The model under review builds one solid part; all positions refer to its coordinate system, in mm. Face numbers are marked on the shaded views. A direction names the side the tool comes from. Coordinates: 2 decimals unless noted, no trailing zeros. Order: outer loops, then holes, each group sorted by start corner. A loop starts at its lowest first (then second) coordinate and runs counter-clockwise, first axis right, second up. Notation, with made-up numbers: (39.25, 60) -> (65.25, 60) arc R18 cw to (65.25, 93) -> close; hole circle Ø9 at (-27, 26). An arc over 180 degrees is marked (long way). Use one line per item in the form item = value.
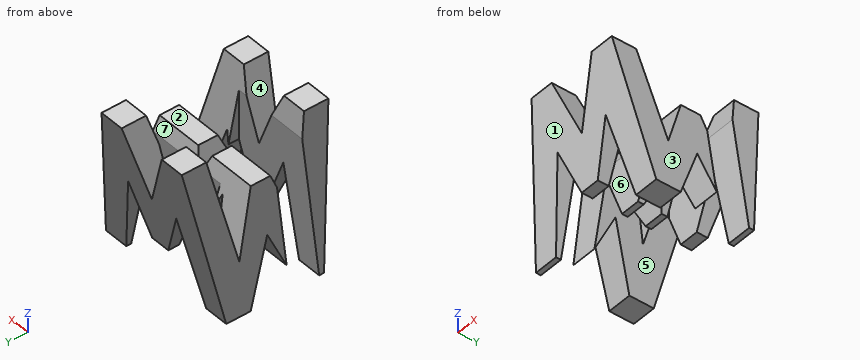
from build123d import *

# Parameters (mm, degrees)
F0_W      = 38.1
F0_H      = 38.1
F1_DEPTH  = 38.1
F6_DEPTH  = 38.1
F8_DEPTH  = 38.1
F9_W      = 25.4
F9_H      = 7.62
F10_DEPTH = 38.1


# Not quite as in the source:
# - a feature names something its author has since deleted; it is built from what else it names


with BuildPart() as f1:
    # F0 (on Front) → F1 (new body)
    with BuildSketch(Plane.XZ):
        with Locations((19.05, 19.05)):
            Rectangle(F0_W, F0_H)
    extrude(amount=F1_DEPTH)

    # F5 (on offset) → F6 (cut)
    with BuildSketch(Plane.YZ.offset(38.1)):
        Polygon((-11.43, 12.2219994664), (-6.35, 38.1), (-31.75, 38.1), (-26.67, 14.2379999161), (-21.59, 27.6940000847), (-16.51, 27.6940000847), align=None)
        Polygon((-31.75, 0), (-38.1, 38.1), (-38.1, 0), align=None)
        Polygon((-25.4, 0), (-19.05, 0), (-19.05, 14.9940000847), align=None)
        Polygon((-19.05, 0), (-12.7, 0), (-19.05, 14.9940000847), align=None)
        Polygon((-6.35, 0), (0, 0), (0, 38.1), align=None)
    extrude(amount=-F6_DEPTH, mode=Mode.SUBTRACT)

    # F7 (on offset) → F8 (cut)
    with BuildSketch(Plane.XZ.offset(38.1)):
        Polygon((0, 38.1), (0, 0), (6.35, 38.1), align=None)
        Polygon((25.4, 38.1), (12.7, 38.1), (19.05, 22.225), align=None)
        Polygon((31.75, 38.1), (38.1, 0), (38.1, 38.1), align=None)
        Polygon((11.340001598, 22.225), (6.35, 0), (31.660001598, 0), (26.580001598, 22.2758815411), (21.500001598, 9.525), (16.420001598, 9.525), align=None)
    extrude(amount=-F8_DEPTH, mode=Mode.SUBTRACT)

    # F9 (on offset) → F10 (cut)
    with BuildSketch(Plane.XY.offset(38.1)):
        with Locations((25.4, -11.43)):
            Rectangle(F9_W, F9_H)
        with Locations((12.7, -26.67)):
            Rectangle(F9_W, F9_H)
    extrude(amount=-F10_DEPTH, mode=Mode.SUBTRACT)


solid = f1.part
Item 1: We need section B-B (z = 23). State how many separate pieces and enclosed holes the cut face has, plus the area to 3 significant figures.
Results found:
separate_pieces = 6
enclosed_holes = 0
area = 571 mm²
Item 2: We need section D-D (z = 33.5). Write out the cut boundary in (x, y).
Results found:
outline = (5.58, -37.33) -> (14.54, -37.33) -> (14.54, -30.77) -> (5.58, -30.77) -> close; (5.58, -7.25) -> (14.54, -7.25) -> (14.54, -0.77) -> (5.58, -0.77) -> close; (23.56, -37.33) -> (32.52, -37.33) -> (32.52, -30.77) -> (23.56, -30.77) -> close; (23.56, -7.25) -> (32.52, -7.25) -> (32.52, -0.77) -> (23.56, -0.77) -> close
Item 3: We need section A-A (x = 3.5). Write out the cut boundary in (y, z).
Results found:
outline = (-35.25, 21) -> (-31.75, 0) -> (-30.48, 0) -> (-30.48, 21) -> close; (-22.86, 6) -> (-19.05, 14.99) -> (-12.7, 0) -> (-6.35, 0) -> (-2.85, 21) -> (-9.71, 21) -> (-11.43, 12.22) -> (-14.31, 21) -> (-22.86, 21) -> close
Item 4: Draft analysis for pull direction Y (two halves, no side actions). For the marked faces 1, 2 and 3, state which applies: released by +Y, released by -Y, zero draft, split by the parting line, or undercut.
Results found:
face_1 = released by -Y
face_2 = undercut
face_3 = zero draft
Item 5: To check wall thickness, follow L1, parallel to Y at x = 31.5, z = 13; L2, parallel to X at y = -7, z = 12.5; L3, parallel to Y at x = 5, z = 23.5. State the ranges of each line that lie inside material, in increasing order. Write a range as from..to.
Results found:
L1 = -33.92..-19.89, -18.21..-15.24, -7.62..-4.18
L2 = 2.08..9.16, 15.23..22.69, 28.81..36.02
L3 = -35.67..-30.48, -22.86..-15.13, -9.22..-2.43
Item 6: Clearance check with flat-ended pins moving along their axes: pin 1 (4 mm diameter, centred on x = 10.5, y = -19.5, fed in from +Z); pin 2 (14.5 mm diameter, centred on x = 21.5, z = 10.5, fed in from +Y); pin 3 (20.5 mm diameter, centred on x = 24.5, z = 13.5, fed in from -Y); pin 4 (1 mm diameter, centred on x = 13.5, z = 10.5, fed in from +Y). State where each tip first meets the part, or that it passes through.
Results found:
pin_1 = 27.69
pin_2 = -3.39
pin_3 = -35.71
pin_4 = through
Item 7: We need section C-C (x = 27.5). Write out the cut boundary in (y, z).
Results found:
outline = (-38.1, 38.1) -> (-34.79, 18.24) -> (-27.52, 18.24) -> (-31.75, 38.1) -> close; (-25.16, 18.24) -> (-15.24, 18.24) -> (-15.24, 23.83) -> (-16.51, 27.69) -> (-21.59, 27.69) -> close; (-7.62, 18.24) -> (-3.31, 18.24) -> (0, 38.1) -> (-6.35, 38.1) -> (-7.62, 31.63) -> close
Item 8: Tool access review of the marked faces 4, 5, 6 and 7: name each direction out of +Z, -Z, +X, -X, +Y, -Y from which nothing blocks a thin tool from reaching the whole face with its end or side.
Results found:
face_4 = +Z, +Y, -Y
face_5 = -Z, +Y, -Y
face_6 = +Z, -Z, -X
face_7 = +Z, +X, -X
